Read the model definition and answer for the solid it produces. Units are mm, in the model's axes. Coordinates: 2 decimals unless noted, no trailing zeros. Order: outer loops, then holes, each group sorted by start corner. A loop starts at its lowest first (then second) coordinate and runs counter-clockwise, first axis right, second up. Notation, with made-up numbers: (3, -33) - (27, -33) arc R25 ccw to (27, 2) - close; hole circle Ø1 at (11, 66). An arc over 180 degrees is marked (long way). Write item = value, one per line.
from build123d import *

# Parameters (mm, degrees)
F1_DEPTH  = 38.1
F3_DEPTH  = 18.542
F5_DEPTH  = 18.796
F6_R      = 3.6195
F7_DEPTH  = 24.257
F9_DEPTH  = 18.796
F11_DEPTH = 19.05


with BuildPart() as f1:
    # F0 (on Top) → F1 (new body)
    with BuildSketch(Plane.XY):
        Polygon((-12.0983748909, -20.955), (12.0983748909, -20.955), (24.1967497817, 0), (12.0983748909, 20.955), (-12.0983748909, 20.955), (-24.1967497817, 0), align=None)
    extrude(amount=F1_DEPTH)

    # F2 (on face) → F3 (cut)
    with BuildSketch(Plane.XY.offset(38.1)):
        Polygon((-11.365140049, -19.685), (11.365140049, -19.685), (22.730280098, 0), (11.365140049, 19.685), (-11.365140049, 19.685), (-22.730280098, 0), align=None)
    extrude(amount=-F3_DEPTH, mode=Mode.SUBTRACT)

    # F4 (on face) → F5 (join)
    with BuildSketch(Plane.XY.offset(38.1)):
        with BuildLine():
            ThreePointArc((-4.692702988, 19.685), (3.4793300822, 16.3000330702), (6.864297012, 8.128))
            ThreePointArc((6.864297012, 8.128), (-7.683874715, -3.0352047683), (-14.7013585559, 13.9065000408))
            Line((-14.7013585559, 13.9065000408), (-22.730280098, 0))
            Line((-22.730280098, 0), (-13.1982271906, -16.509999936))
            ThreePointArc((-13.1982271906, -16.509999936), (-9.3424667403, -7.2013709935), (-1.3489658396, -13.335))
            ThreePointArc((-1.3489658396, -13.335), (-3.2088377669, -17.8251280484), (-7.6989658052, -19.685))
            Line((-7.6989658052, -19.685), (7.6989658396, -19.685))
            ThreePointArc((7.6989658396, -19.685), (3.2088377791, -8.8448719395), (14.0489658396, -13.335))
            ThreePointArc((14.0489658396, -13.335), (13.8325948227, -14.9785009883), (13.1982271, -16.510000093))
            Line((13.1982271, -16.510000093), (20.8971929349, -3.1750001012))
            ThreePointArc((20.8971929349, -3.1750001012), (9.0479316793, 1.601e-07), (20.897193095, 3.1749998238))
            Line((20.897193095, 3.1749998238), (11.365140049, 19.685))
            Line((11.365140049, 19.685), (-4.692702988, 19.685))
        make_face()
        with BuildLine():
            ThreePointArc((-7.6989658052, -19.685), (-10.8739658568, -18.8342613042), (-13.1982271906, -16.509999936))
            Line((-13.1982271906, -16.509999936), (-11.365140049, -19.685))
            Line((-11.365140049, -19.685), (-7.6989658052, -19.685))
        make_face()
        with BuildLine():
            Line((11.365140049, -19.685), (13.1982271, -16.510000093))
            ThreePointArc((13.1982271, -16.510000093), (10.8739657932, -18.8342613409), (7.6989658396, -19.685))
            Line((7.6989658396, -19.685), (11.365140049, -19.685))
        make_face()
        with BuildLine():
            Line((22.730280098, 0), (20.897193095, 3.1749998238))
            ThreePointArc((20.897193095, 3.1749998238), (21.5315607026, 1.6435008381), (21.7479316793, 0))
            ThreePointArc((21.7479316793, 0), (21.5315606611, -1.6435009928), (20.8971929349, -3.1750001012))
            Line((20.8971929349, -3.1750001012), (22.730280098, 0))
        make_face()
        with BuildLine():
            ThreePointArc((-14.7013585559, 13.9065000408), (-10.4712029675, 18.1366556033), (-4.692702988, 19.685))
            Line((-4.692702988, 19.685), (-11.365140049, 19.685))
            Line((-11.365140049, 19.685), (-14.7013585559, 13.9065000408))
        make_face()
    extrude(amount=-F5_DEPTH)

    # F6 (on face) → F7 (cut)
    with BuildSketch(Plane.XY.offset(38.1)):
        with Locations((-4.914952988, 8.512948292)):
            Circle(F6_R)
    extrude(amount=-F7_DEPTH, mode=Mode.SUBTRACT)

    # F8 (on face) → F9 (join)
    with BuildSketch(Plane(origin=(0, 0, 0), x_dir=(1, 0, 0), z_dir=(0, 0, -1))):
        Polygon((-20.1272964094, -11.6205), (-18.1475623363, -10.4775), (-19.2905623363, -8.4977659269), (-21.8417964094, -8.6508988904), align=None)
        Polygon((-17.0045623363, -12.4572340731), (-18.1475623363, -10.4775), (-20.1272964094, -11.6205), (-18.4127964094, -14.5901011096), align=None)
    extrude(amount=-F9_DEPTH)

    # F10 (on face) → F11 (cut)
    with BuildSketch(Plane(origin=(0, 0, 0), x_dir=(1, 0, 0), z_dir=(0, 0, -1))):
        Polygon((-2.54, -20.955), (0, -20.955), (0, -18.415), (-3.81, -18.415), align=None)
        Polygon((0, -18.415), (0, -20.955), (2.54, -20.955), (3.81, -18.415), align=None)
    extrude(amount=-F11_DEPTH, mode=Mode.SUBTRACT)


solid = f1.part
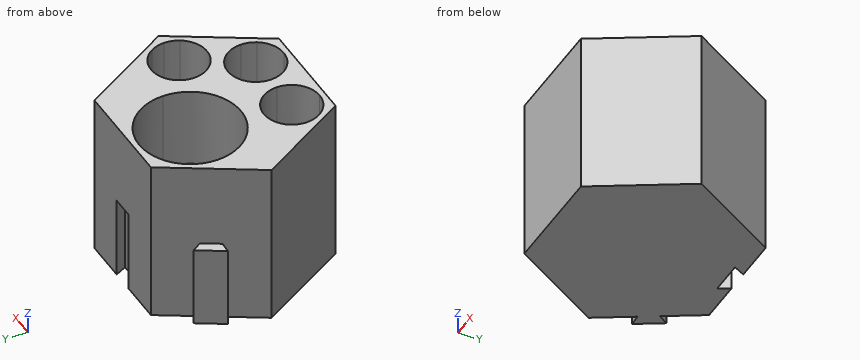
1) The part is cut by section D-D (z = 11). Determine the outline of the cut face in (x, y) (3 decimals).
Returned:
outline = (-24.197, 0) - (-12.098, -20.955) - (12.098, -20.955) - (24.197, 0) - (12.098, 20.955) - (2.54, 20.955) - (3.81, 18.415) - (-3.81, 18.415) - (-2.54, 20.955) - (-12.098, 20.955) - (-17.005, 12.457) - (-18.413, 14.59) - (-21.842, 8.651) - (-19.291, 8.498) - close
2) Flat-ended cylindrical pins translate along their axes: pin 1 Ø6 at (y, z) = (-12.5, 8.5) entering from +X; pin 2 Ø1.5 at (x, z) = (-17.5, 7.5) entering from +Y; pin 3 Ø4 at (y, z) = (-15.5, 31.5) entering from +X. Find the tip coordinate at first contact, or state that the pin passes through.
Returned:
pin_1 = 18.71
pin_2 = 14.34
pin_3 = 16.4
3) The part is cut by section A-A (z = 33.5). Count the separate pieces of the cut face and the enclosed holes in it, and give its area (3 significant figures).
Returned:
separate_pieces = 1
enclosed_holes = 4
area = 721 mm^2
4) Straight lines are drawn through the part: line 1 along Y through (x, z) = (11, 35.5) (3 decimals); line 2 along X through (y, z) = (-18, 26.5); line 3 along Y through (x, z) = (13, 24). For each, find the intervals that lie inside material, in ascending order. Write a range as from..to.
Returned:
line_1 = -20.955..-18.76, -7.91..-4.58, 4.58..20.955
line_2 = -13.8..-12.01, -3.39..3.39, 12.01..13.8
line_3 = -19.39..-16.83, -9.84..-5.88, 5.88..19.39
5) The part is cut by section B-B (z = 15.5). Determine the outline of the cut face in (x, y) (1 decimal), and give its area (3 significant figures).
Returned:
outline = (-24.2, 0) - (-12.1, -21) - (12.1, -21) - (24.2, 0) - (12.1, 21) - (2.5, 21) - (3.8, 18.4) - (-3.8, 18.4) - (-2.5, 21) - (-12.1, 21) - (-17, 12.5) - (-18.4, 14.6) - (-21.8, 8.7) - (-19.3, 8.5) - close; hole circle Ø7.2 at (-4.9, 8.5)
area = 1,480 mm^2
6) The part is cut by section C-C (y = 1.5). Determine the outline of the cut face in (x, z).
Returned:
outline = (-23.33, 0) - (23.33, 0) - (23.33, 38.1) - (21.57, 38.1) - (21.57, 19.56) - (9.23, 19.56) - (9.23, 38.1) - (4.77, 38.1) - (4.77, 19.56) - (-14.16, 19.56) - (-14.16, 38.1) - (-23.33, 38.1) - close
